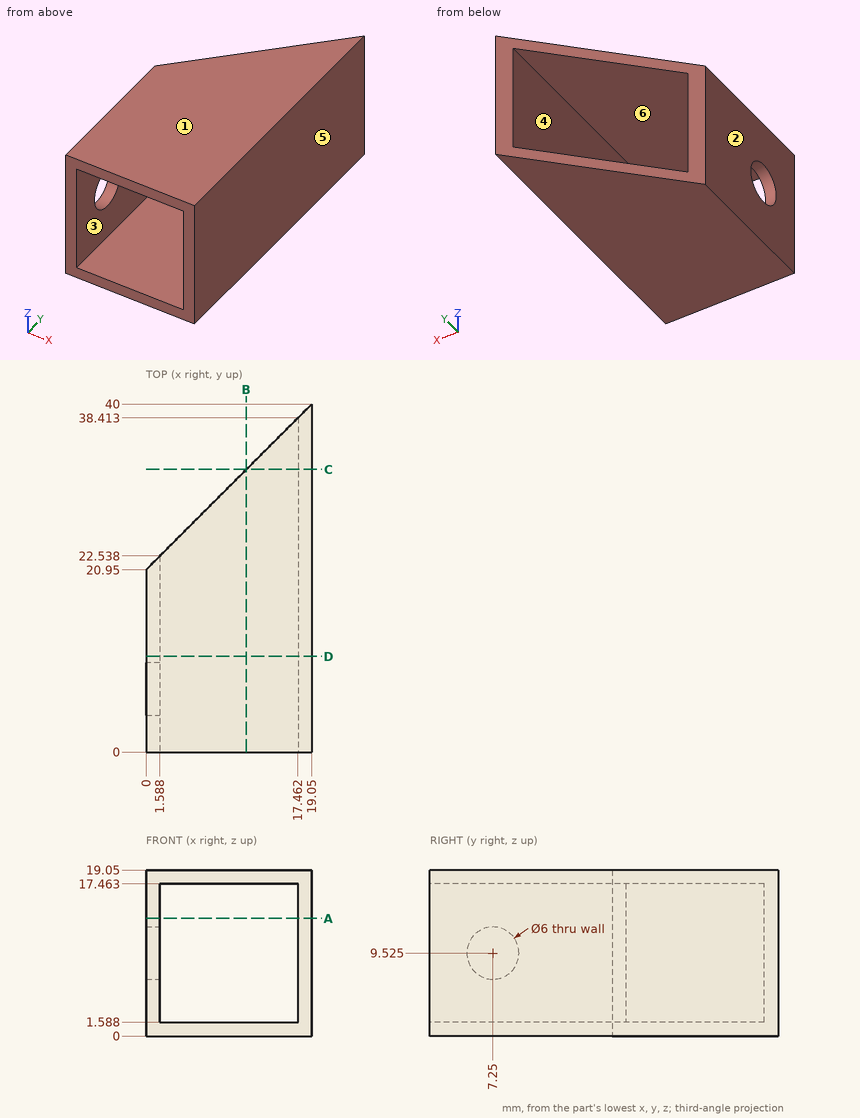
Can you work these out from the drawing? Everything is in mm from the part's minimum corner. A direction names the side the tool comes from. Coordinates: 2 decimals unless noted, no trailing zeros. Loops run counter-clockwise (first coordinate to the right, second up) from the corner with the lowest first, then second, coordinate; pieces in that order, holes last.
1. Imagine slicing it at C-C, the plane y = 32.5. Please give me the cut outline in (x, z).
2. For the marked faces 5 and 6, which set-ups out of +Z, -Z, +X, -X, +Y, -Y let a thin tool reach every point of the face, with its end or its side?
3. I need wall thicknesses on L1, parallel to Z at x = 14.75, y = 29; L2, parallel to X at y = 34, z = 7. Which ranges of each line are inside material? Lowest first, please.
4. Imagine slicing it at B-B, the plane x = 11.5. Please give me the cut outline in (y, z), and give its area (3 significant figures).
5. If we mould it in two halves opening along X, with no side actions, what happens to the marked faces 1, 2, 3 and 4? For each: pulls with the +X half, pulls with the -X half, needs draft (parallel to the pull), parting line crosses it, or undercut.
6. Imagine slicing it at A-A, the plane z = 13.5. Please give me the cut outline in (x, y).
7. For P1, Ø5, axis at x = 11.5, z = 17, coming from the +Y side (1 decimal); P2, Ø1, axis at x = 2, z = 7, coming from the +Y side; P3, Ø1, axis at x = 4, z = 13, coming from the -Y side; P4, Ø6, axis at y = 30.5, z = 3, coming from the -X side (1 decimal), each with a flat end and sliding along its axis, tell me the tip position at first contact or that it passes through.
8. Imagine slicing it at D-D, the plane y = 11. Please give me the cut outline in (x, z).
Taken from the geometry:
1. outline: (11.55, 0) - (19.05, 0) - (19.05, 19.05) - (11.55, 19.05) - (11.55, 17.46) - (17.46, 17.46) - (17.46, 1.59) - (11.55, 1.59) - close
2. face 5: +Z, -Z, +X, +Y, -Y
2. face 6: +Y, -Y
3. L1: z = 0 to 1.59, 17.46 to 19.05
3. L2: x = 17.46 to 19.05
4. outline: (0, 0) - (32.45, 0) - (32.45, 1.59) - (0, 1.59) - close; (0, 17.46) - (32.45, 17.46) - (32.45, 19.05) - (0, 19.05) - close
4. area: 103 mm2
5. face 1: needs draft
5. face 2: pulls with the -X half
5. face 3: undercut
5. face 4: undercut
6. outline: (0, 0) - (1.59, 0) - (1.59, 22.54) - (0, 20.95) - close; (17.46, 0) - (19.05, 0) - (19.05, 40) - (17.46, 38.41) - close
7. P1: stops at y = 34.9
7. P2: stops at y = 22.54
7. P3: passes through
7. P4: stops at x = 6.9
8. outline: (0, 0) - (19.05, 0) - (19.05, 19.05) - (0, 19.05) - close; hole (1.59, 1.59) - (17.46, 1.59) - (17.46, 17.46) - (1.59, 17.46) - close
